```python
from build123d import *


with BuildPart() as f1:
    # F0 (on Front) → F1 (revolve)
    with BuildSketch(Plane.XZ):
        with BuildLine():
            Line((0, 27.94), (0, 0))
            Line((0, 0), (13.335, 0))
            Line((13.335, 0), (13.335, 27.94))
            Line((13.335, 27.94), (15.875, 27.94))
            ThreePointArc((15.875, 27.94), (17.494737, 28.793452), (18.706733, 30.165673))
            Line((18.706733, 30.165673), (28.448, 104.483135))
            ThreePointArc((28.448, 104.483135), (25.00778, 119.412812), (11.573426, 126.77817))
            Line((11.573426, 126.77817), (9.020732, 126.983041))
            ThreePointArc((9.020732, 126.983041), (5.100598, 130.287789), (0, 130.81))
            Line((0, 130.81), (0, 27.94))
        make_face()
    revolve(axis=Axis((0, 0, 65.405), (0, 0, 1)))


solid = f1.part
```
For this review, take the finished solid that the model builds, in its own axes (mm). Round coordinates to 2 decimals unless told otherwise and drop trailing zeros. Loops run counter-clockwise (first coordinate to the right, second up) from the corner with the lowest first, then second, coordinate; pieces in that order, holes last.
(1) We need section B-B (z = 67.5). Give the boundary of the cut face in (x, y).
Returned:
outline: circle Ø47.2 at (0, 0)
(2) Mouldability with a two-part tool opening along X and no side actions: class faces 1 (the flat face through (0, 0, 0)), 2 (the cylindrical face through (-1.74, 13.22, 14.17)) as released by +X, released by -X, zero draft, split by the parting line, or undercut.
Returned:
face 1: zero draft
face 2: split by the parting line
(3) Clearance check with flat-ended pins moving along their axes: P1, Ø3, axis at x = 2.5, z = 103, coming from the -Y side; P2, Ø8, axis at y = 9, z = 30, coming from the +X side; P3, Ø1.5, axis at y = 14, z = 100.5, coming from the -X side. State where each tip first meets the part, or that it passes through.
Returned:
P1: stops at y = -28.37
P2: stops at x = 18.13
P3: stops at x = -24.6
(4) We need section A-A (z = 53.5). Give the boundary of the cut face in (x, y).
Returned:
outline: circle Ø43.53 at (0, 0)
(5) Wall thickness on line 1 along Y through (x, z) = (5.5, 17); line 2 along Z through (x, y) = (-14.5, -11); line 3 along Y through (x, z) = (-10.5, 82): over which ranges is each line inside the solid? List them lowest first.
Returned:
line 1: y = -12.15 to 12.15
line 2: z = 29.47 to 124.98
line 3: y = -23.24 to 23.24
